For this review, take the finished solid that the model builds, in its own axes (mm). A direction names the side the tool comes from. Give positions to 0.01 mm unless a question says otherwise; leave off trailing zeros. Loops run counter-clockwise (first coordinate to the right, second up) from the corner with the lowest first, then second, coordinate; pieces in that order, holes last.
Solid Edge part; units mm, degrees
sketch "Sketch1" plane through (0, 0, 0) normal (0, -1, 0) x (1, 0, 0)
  line L0 (-2.5, -1) -> (2.5, -1)
  line L1 (2.5, -1) -> (2.5, 1)
  line L2 (2.5, 1) -> (-2.5, 1)
  line L3 (-2.5, 1) -> (-2.5, -1)
extrude "Protrusion1" add sketch "Sketch1" along normal mid plane 20
fillet "Round_2" radius 2.5 4 edges at (-2.5, -10, 0) (2.5, -10, 0) (2.5, 10, 0) (-2.5, 10, 0)
hole "Hole_2" at (0, -7.5, 1) direction (0, 0, -1) diameter 2.6 end through all
hole "Hole_4" at (0, 7.5, 1) direction (0, 0, -1) diameter 1.5 end through all
sketch "Sketch2" plane through (0, 0, 1) normal (0, 0, 1) x (0, 1, 0)
  circle A0 centre (-7.5, 0) radius 2.5
  circle A1 centre (-7.5, 0) radius 1.3
extrude "ExtrudedProtrusion_2" add sketch "Sketch2" along normal blind 3
properties material "ABS Plastic, high impact"
Item 1: Take a section at B-B on x = 2.1. Give the boundary of the cut face in (y, z), and give its area (3 significant figures).
Answer:
outline: (-8.86, -1) - (8.86, -1) - (8.86, 1) - (-6.14, 1) - (-6.14, 4) - (-8.86, 4) - close
area: 43.6 mm2
Item 2: Take a section at A-A on z = 0.65. State how many separate pieces and enclosed holes the cut face has, and give its area (3 significant figures).
Answer:
separate pieces: 1
enclosed holes: 2
area: 87.6 mm2
Item 3: Take a section at C-C on x = -0.35. Give the boundary of the cut face in (y, z).
Answer:
outline: (-9.98, -1) - (-8.75, -1) - (-8.75, 4) - (-9.98, 4) - close; (-6.25, -1) - (6.84, -1) - (6.84, 1) - (-5.02, 1) - (-5.02, 4) - (-6.25, 4) - close; (8.16, -1) - (9.98, -1) - (9.98, 1) - (8.16, 1) - close
Item 4: Take a section at D-D on z = 3.4. Give the boundary of the cut face in (x, y).
Answer:
outline: circle Ø5 at (0, -7.5); hole circle Ø2.6 at (0, -7.5)
Item 5: Clearance check with flat-ended pins moving along their axes: pin 1 Ø3 at (x, y) = (0, -7.5) entering from +Z; pin 2 Ø1.5 at (x, y) = (0, 2) entering from +Z. State where each tip first meets the part, or that it passes through.
Answer:
pin 1: stops at z = 4
pin 2: stops at z = 1
Item 6: Tool access review of faces 1 (the cylindrical face through (0, -10, 2)), 2 (the cylindrical face through (2, -9, 0)): name each direction out of +Z, -Z, +X, -X, +Y, -Y from which nothing blocks a thin tool from reaching the whole face with its end or side.
Answer:
face 1: +Z
face 2: +Z, -Z, +X, -Y
Item 7: For L1, parallel to Y at x = 0, z = 0.05; L2, parallel to X at y = 7.5, z = -0.25; L3, parallel to Y at x = 0, z = 3.3, list the stretches that pass through material, from the lowest coordinate up.
Answer:
L1: y = -10 to -8.8, -6.2 to 6.75, 8.25 to 10
L2: x = -2.5 to -0.75, 0.75 to 2.5
L3: y = -10 to -8.8, -6.2 to -5
Item 8: The part is to be moulded in two halves that separate along X. For faces 3 (the flat face through (0, 0, -1)), 4 (the cylindrical face through (-2, 9, 0)), 5 (the cylindrical face through (0.03, 8.25, 0.01)), say which applies: released by +X, released by -X, zero draft, split by the parting line, or undercut.
Answer:
face 3: zero draft
face 4: released by -X
face 5: undercut
